Autodesk Inventor part; units mm, degrees
ref_plane "YZ Plane" through (0, 0, 0) normal (1, 0, 0) x (0, 1, 0)
ref_plane "XZ Plane" through (0, 0, 0) normal (0, 1, 0) x (-1, 0, 0)
ref_plane "XY Plane" through (0, 0, 0) normal (0, 0, 1) x (1, 0, 0)
sketch "Sketch1" plane through (0, 0, 0) normal (0, 0, 1) x (1, 0, 0)
  line L0 (0, 36.15) -> (10, 36.15)
  line L1 (10, 36.15) -> (10, 47.9)
  line L2 (10, 47.9) -> (90.4, 47.9)
  line L3 (90.4, 47.9) -> (90.4, -47.9)
  line L4 (90.4, -47.9) -> (2, -47.9)
  line L5 (10, -15.15) -> (0, -15.15)
  line L6 (-5.5, 48) -> (90.5, 48) construction
  line L7 (90.5, 48) -> (90.5, -48) construction
  line L8 (90.5, -48) -> (-5.5, -48) construction
  line L9 (-5.5, -48) -> (-5.5, 48) construction
  line L10 (-5.4, 47.9) -> (-3.4, 47.9) construction
  line L11 (-3.4, 47.9) -> (-3.4, -47.9) construction
  line L12 (-3.4, -47.9) -> (-5.4, -47.9) construction
  line L13 (-5.4, -47.9) -> (-5.4, 47.9) construction
  line L14 (-3.4, 38.5) -> (7.85, 38.5) construction
  line L15 (7.85, 38.5) -> (7.85, -17.5) construction
  line L16 (7.85, -17.5) -> (-3.4, -17.5) construction
  line L17 (-3.4, -17.5) -> (-3.4, 38.5) construction
  line L18 (2, -47.9) -> (2, -18.65)
  line L19 (2, -18.65) -> (10, -18.65)
  arc A0 (10, -18.65) -> (10, -15.15) centre (10, -16.9) ccw
  line L20 (0, 24) -> (90.5, 24) construction
  circle A1 centre (-2.5, 47.1) radius 0.9 construction
  circle A2 centre (-0.7, 47.1) radius 0.9 construction
  circle A3 centre (1.1, 47.1) radius 0.9 construction
  circle A4 centre (2.9, 47.1) radius 0.9 construction
  circle A5 centre (4.7, 47.1) radius 0.9 construction
  circle A6 centre (6.5, 47.1) radius 0.9 construction
  circle A7 centre (8.3, 47.1) radius 0.9 construction
  circle A8 centre (-2.5, 45.3) radius 0.9 construction
  circle A9 centre (-0.7, 45.3) radius 0.9 construction
  circle A10 centre (1.1, 45.3) radius 0.9 construction
  circle A11 centre (2.9, 45.3) radius 0.9 construction
  circle A12 centre (4.7, 45.3) radius 0.9 construction
  circle A13 centre (6.5, 45.3) radius 0.9 construction
  circle A14 centre (8.3, 45.3) radius 0.9 construction
  circle A15 centre (-2.5, 43.5) radius 0.9 construction
  circle A16 centre (-0.7, 43.5) radius 0.9 construction
  circle A17 centre (1.1, 43.5) radius 0.9 construction
  circle A18 centre (2.9, 43.5) radius 0.9 construction
  circle A19 centre (4.7, 43.5) radius 0.9 construction
  circle A20 centre (6.5, 43.5) radius 0.9 construction
  circle A21 centre (8.3, 43.5) radius 0.9 construction
  circle A22 centre (-2.5, 41.7) radius 0.9 construction
  circle A23 centre (-0.7, 41.7) radius 0.9 construction
  circle A24 centre (1.1, 41.7) radius 0.9 construction
  circle A25 centre (2.9, 41.7) radius 0.9 construction
  circle A26 centre (4.7, 41.7) radius 0.9 construction
  circle A27 centre (6.5, 41.7) radius 0.9 construction
  circle A28 centre (8.3, 41.7) radius 0.9 construction
  circle A29 centre (-2.5, 39.9) radius 0.9 construction
  circle A30 centre (-0.7, 39.9) radius 0.9 construction
  circle A31 centre (1.1, 39.9) radius 0.9 construction
  circle A32 centre (2.9, 39.9) radius 0.9 construction
  circle A33 centre (4.7, 39.9) radius 0.9 construction
  circle A34 centre (6.5, 39.9) radius 0.9 construction
  circle A35 centre (8.3, 39.9) radius 0.9 construction
  line L21 (0, 36.15) -> (0, 24.95)
  line L22 (0, 24.95) -> (8.4, 24.95)
  arc A36 (8.4, 23.05) -> (8.4, 24.95) centre (8.4, 24) ccw
  line L23 (8.4, 23.05) -> (0, 23.05)
  line L24 (0, 23.05) -> (0, -15.15)
  point P0 (0, 0)
  point P1 (-5.5, 0)
  point P2 (90.4, 0)
  point P3 (90.5, 0)
  dimension "d0" = 51.3
  dimension "d1" = 95.8
  dimension "d3" = 10
  dimension "d20" = 96
  dimension "d21" = 96
  dimension "d22" = 0.1
  dimension "d23" = 0.1
  dimension "d24" = 2
  dimension "d25" = 0.1
  dimension "d28" = 11.25
  dimension "d29" = 56
  dimension "d31" = 9.5
  dimension "d32" = 30.5
  dimension "d34" = 3.5
  dimension "d35" = 12.15
  dimension "d36" = 39.15
  dimension "d37" = 14.5
  dimension "d38" = 1.15
  dimension "d39" = 1.8
  dimension "d42" = 1.8
  dimension "d45" = 1.8
  dimension "d48" = 2
  dimension "d49" = 3.4
  dimension "d50" = 1.9
  dimension "d51" = 8.4
  dimension "d52" = 24
extrude "Extrusion1" add sketch "Sketch1" along normal mid plane 1.6
chamfer "Chamfer1" distance 0.5 angle 45 4 edges at (0, 36.15, 0) (0, 24.95, 0) (0, 23.05, 0) (0, -15.15, 0)
fillet "Fillet1" radius 0.5 6 edges at (10, 36.15, 0) (10, 47.9, 0) (90.4, 47.9, 0) (90.4, -47.9, 0) (2, -47.9, 0) (2, -18.65, 0)
equation "\"d23\" = d22"
equation "\"d25\" = d22"
equation "\"d42\" = d39"
equation "\"d45\" = d39"
properties part number "CardStandard" material "Epoxy Resin"
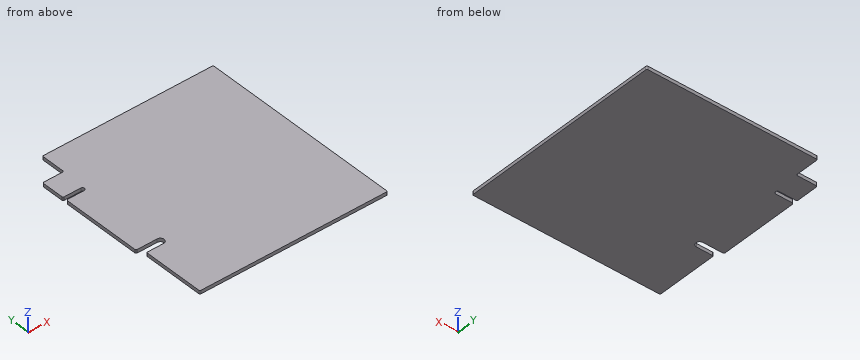
Check sheet for the modelled part. Datum: model origin and axes. Units: mm. Round coordinates to 2 decimals unless told otherwise and drop trailing zeros. Loops run counter-clockwise (first coordinate to the right, second up) from the corner with the lowest first, then second, coordinate; pieces in that order, holes last. Notation, with made-up numbers: (52.5, 16) -> (81.5, 16) arc R18 ccw to (81.5, 31) -> close; hole circle Ø6 at (58.5, 34). An arc over 180 degrees is marked (long way). Answer in a Markdown table with one row per item.
Q1. Sectioned sample at A-A on z = -0.45. Enter the section's corners in (x, y).
Data:
| item | result |
|---|---|
| outline | (0, -14.65) -> (0.5, -15.15) -> (10, -15.15) arc R1.75 cw to (10, -18.65) -> (2.5, -18.65) arc R0.5 ccw to (2, -19.15) -> (2, -47.4) arc R0.5 ccw to (2.5, -47.9) -> (89.9, -47.9) arc R0.5 ccw to (90.4, -47.4) -> (90.4, 47.4) arc R0.5 ccw to (89.9, 47.9) -> (10.5, 47.9) arc R0.5 ccw to (10, 47.4) -> (10, 36.65) arc R0.5 cw to (9.5, 36.15) -> (0.5, 36.15) -> (0, 35.65) -> (0, 25.45) -> (0.5, 24.95) -> (8.4, 24.95) arc R0.95 cw to (8.4, 23.05) -> (0.5, 23.05) -> (0, 22.55) -> close |
Q2. Go/stop test with flat-tipped pins: P1, Ø0.8, axis at y = -31, z = -0.5, coming from the -X side; P2, Ø0.5, axis at y = 42, z = 0, coming from the -X side; P3, Ø0.8, axis at x = 4, z = 0.5, coming from the +Y side. Record where each tip stops, or that it passes through.
Data:
| item | result |
|---|---|
| P1 | stops at x = 2 |
| P2 | stops at x = 10 |
| P3 | stops at y = 36.15 |
Q3. Thickness scan on L1, parallel to Y at x = 7, z = 0.6; L2, parallel to X at y = -35, z = -0.35; L3, parallel to X at y = 42.5, z = 0.5. Record the ranges inside material, lowest first.
Data:
| item | result |
|---|---|
| L1 | y = -47.9 to -18.65, -15.15 to 23.05, 24.95 to 36.15 |
| L2 | x = 2 to 90.4 |
| L3 | x = 10 to 90.4 |
Q4. Sectioned sample at B-B on y = -39. Enter the section's corners in (x, z), then the cut area to 3 significant figures.
Data:
| item | result |
|---|---|
| outline | (2, -0.8) -> (90.4, -0.8) -> (90.4, 0.8) -> (2, 0.8) -> close |
| area | 141 mm^2 |
